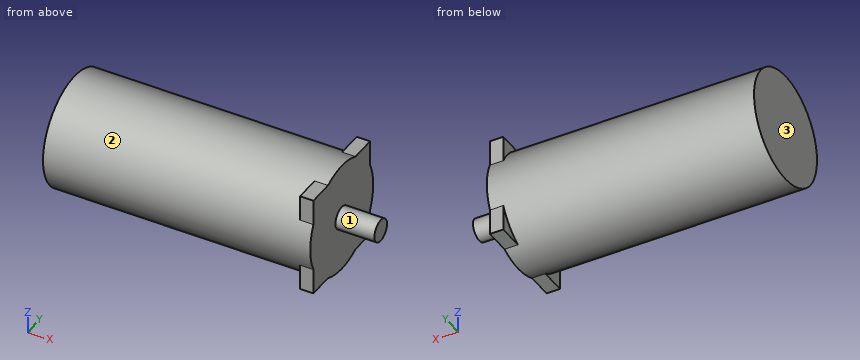
from build123d import *

# Parameters (mm, degrees)
SKETCH1_W           = 90
SKETCH1_H           = 90
BOSS_EXTRUDE1_DEPTH = 12
SKETCH2_R           = 50
BOSS_EXTRUDE2_DEPTH = 240
SKETCH3_R           = 10
BOSS_EXTRUDE3_DEPTH = 35


with BuildPart() as part:
    # Sketch1 → Boss-Extrude1 (new body)
    with BuildSketch(Plane.YZ):
        Rectangle(SKETCH1_W, SKETCH1_H)
    extrude(amount=-BOSS_EXTRUDE1_DEPTH)

    # Sketch2 → Boss-Extrude2 (add)
    with BuildSketch(Plane.YZ):
        with Locations(Location((0, 0, 0), (0, 0, 270))):
            Circle(SKETCH2_R)
    extrude(amount=-BOSS_EXTRUDE2_DEPTH)

    # Sketch3 → Boss-Extrude3 (add)
    with BuildSketch(Plane(origin=(0, 0, 0), x_dir=(0, 0, -1), z_dir=(1, 0, 0))):
        with Locations(Location((0, 0, 0), (0, 0, 180))):
            Circle(SKETCH3_R)
    extrude(amount=BOSS_EXTRUDE3_DEPTH)


solid = part.part
Could you check a few things on this model? Use its own coordinates, in mm. Face numbers are marked on the shaded views. A direction names the side the tool comes from. Coordinates: 2 decimals unless noted, no trailing zeros. Order: outer loops, then holes, each group sorted by start corner. A loop starts at its lowest first (then second) coordinate and runs counter-clockwise, first axis right, second up. Notation, with made-up numbers: (57, 32.25) -> (67, 32.25) arc R35 cw to (67, 70.25) -> close; hole circle Ø1 at (-29.5, 45.5). An arc over 180 degrees is marked (long way). One line per question, with ' | ' between items.
Q1. I'm going to push flat-ended pins straight in: P1, Ø13, axis at x = -5.5, y = -35, coming from the -Z side; P2, Ø13, axis at x = -7, z = 39, coming from the -Y side; P3, Ø6, axis at x = -205, z = -2, coming from the +Y side. Where does each tip first touch, or does it pass through?
Return value:
P1: z = -45 | P2: y = -45 | P3: y = 50
Q2. On a 3-axis mill with a long thin cutter (end or side, diameter ignored), from which of +Z, -Z, +X, -X, +Y, -Y can I reach the whole of each face in a straight line? I mean the marked faces 1, 2 and 3. Say none if no direction works.
Return value:
face 1: +X | face 2: -X | face 3: +Z, -Z, -X, +Y, -Y
Q3. Imagine slicing it at C-C on x = -127. Please give me the cut outline in (y, z), and give its area (3 significant figures).
Return value:
outline: circle Ø100 at (0, 0) | area: 7,850 mm²
Q4. If I drill on L1, parallel to X at y = 28.5, z = 27.5; L2, parallel to Z at x = -38.5, y = 32; L3, parallel to Z at x = -210, y = -25, over which ranges is the centre line in solid material (lowest first)?
Return value:
L1: -240 to 0 | L2: -38.42 to 38.42 | L3: -43.3 to 43.3
Q5. Imagine slicing it at A-A on z = 0. Please give me the cut outline in (x, y), and give its area (3 significant figures).
Return value:
outline: (-240, -50) -> (0, -50) -> (0, -10) -> (35, -10) -> (35, 10) -> (0, 10) -> (0, 50) -> (-240, 50) -> close | area: 24,700 mm²
